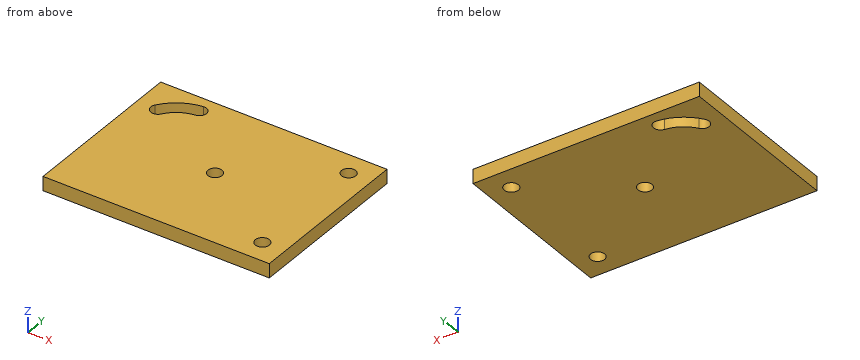
from build123d import *

# Parameters (mm, degrees)
SKETCH1_W           = 80
SKETCH1_H           = 60
SKETCH1_R           = 2.5
BOSS_EXTRUDE1_DEPTH = 5
SKETCH2_R           = 2.5
CUT_EXTRUDE1_DEPTH  = 6


with BuildPart() as part:
    # Sketch1 → Boss-Extrude1 (new body)
    with BuildSketch(Plane.XY):
        with Locations((40, -30)):
            Rectangle(SKETCH1_W, SKETCH1_H)
        with Locations((40, -30)):
            Circle(SKETCH1_R, mode=Mode.SUBTRACT)
    extrude(amount=BOSS_EXTRUDE1_DEPTH)

    # Sketch2 → Cut-Extrude1 (cut, through all)
    with BuildSketch(Plane.XY.offset(5)):
        with Locations((72, -52)):
            Circle(SKETCH2_R)
        with Locations((72, -8)):
            Circle(SKETCH2_R)
        with BuildLine():
            ThreePointArc((17.552814057, -3.5), (10.699313896, -5.865002188), (5.454493121, -10.87055459))
            ThreePointArc((5.454493121, -10.87055459), (6.127589233, -14.341425031), (9.598459675, -13.66832892))
            ThreePointArc((9.598459675, -13.66832892), (13.300686104, -10.134997812), (18.138450924, -8.465584503))
            ThreePointArc((18.138450924, -8.465584503), (20.328424742, -5.689973818), (17.552814057, -3.5))
        make_face()
    extrude(amount=-CUT_EXTRUDE1_DEPTH, mode=Mode.SUBTRACT)


solid = part.part
Geometry check sheet. Reference: the model listing, model coordinates, mm. Coordinates: 2 decimals unless noted, no trailing zeros. Order: outer loops, then holes, each group sorted by start corner. A loop starts at its lowest first (then second) coordinate and runs counter-clockwise, first axis right, second up. Notation, with made-up numbers: (-15.5, 7.5) -> (18.5, 7.5) arc R27 ccw to (18.5, 45.5) -> close; hole circle Ø7 at (10.25, -39). An arc over 180 degrees is marked (long way). Use a Markdown table: item, result. Add a question column.
1. Cross-section at A-A (x = 72). Enter the section's corners in (y, z).
2. Cross-section at C-C (x = 40). Enter the section's corners in (y, z).
3. Material ranges on L1, parallel to Y at x = 72, z = 3.2; L2, parallel to X at y = -10, z = 4.1; L3, parallel to Y at x = 20, z = 4.25, recorded low to high.
4. Cross-section at B-B (y = -52). Enter the section's corners in (x, z).
5. Cross-section at D-D (z = 1.4). Enter the section's corners in (x, y), and give its area (3 significant figures).
Filled sheet:
| question | item | result |
|---|---|---|
| 1 | outline | (-60, 0) -> (-54.5, 0) -> (-54.5, 5) -> (-60, 5) -> close; (-49.5, 0) -> (-10.5, 0) -> (-10.5, 5) -> (-49.5, 5) -> close; (-5.5, 0) -> (0, 0) -> (0, 5) -> (-5.5, 5) -> close |
| 2 | outline | (-60, 0) -> (-32.5, 0) -> (-32.5, 5) -> (-60, 5) -> close; (-27.5, 0) -> (0, 0) -> (0, 5) -> (-27.5, 5) -> close |
| 3 | L1 | -60 to -54.5, -49.5 to -10.5, -5.5 to 0 |
| 3 | L2 | 0 to 6.08, 13.53 to 70.5, 73.5 to 80 |
| 3 | L3 | -60 to -7.25, -4.71 to 0 |
| 4 | outline | (0, 0) -> (69.5, 0) -> (69.5, 5) -> (0, 5) -> close; (74.5, 0) -> (80, 0) -> (80, 5) -> (74.5, 5) -> close |
| 5 | outline | (0, -60) -> (80, -60) -> (80, 0) -> (0, 0) -> close; hole (5.45, -10.87) arc R2.5 ccw to (9.6, -13.67) arc R12 cw to (18.14, -8.47) arc R2.5 ccw to (17.55, -3.5) arc R17 ccw to start; hole circle Ø5 at (40, -30); hole circle Ø5 at (72, -52); hole circle Ø5 at (72, -8) |
| 5 | area | 4,660 mm2 |
